```python
from build123d import *

# Parameters (mm, degrees)
BOSS_EXTRUDE1_START         = -2.9464
BOSS_EXTRUDE1_OUTLINE_W     = 230
BOSS_EXTRUDE1_OUTLINE_H     = 101.6
BOSS_EXTRUDE1_OUTLINE_R     = 4
BOSS_EXTRUDE1_OUTLINE_W_2   = 15
BOSS_EXTRUDE1_OUTLINE_H_2   = 91.6
BOSS_EXTRUDE1_DEPTH         = 2.9464
BOSS_EXTRUDE1_START_2       = -101.6
BOSS_EXTRUDE1_2_OUTLINE_W   = 200
BOSS_EXTRUDE1_2_OUTLINE_H   = 101.6
BOSS_EXTRUDE1_2_OUTLINE_R   = 4
BOSS_EXTRUDE1_2_OUTLINE_W_2 = 140
BOSS_EXTRUDE1_2_OUTLINE_H_2 = 40
BOSS_EXTRUDE1_2_DEPTH       = 2.9464
BOSS_EXTRUDE1_START_3       = -98.6536
BOSS_EXTRUDE1_3_OUTLINE_W   = 30
BOSS_EXTRUDE1_3_OUTLINE_H   = 2.9464
BOSS_EXTRUDE1_3_DEPTH       = 95.7072
BOSS_EXTRUDE1_4_OUTLINE_W   = 140
BOSS_EXTRUDE1_4_OUTLINE_H   = 2.9464
BOSS_EXTRUDE1_4_DEPTH       = 17.8536
BOSS_EXTRUDE1_START_4       = -20.8
BOSS_EXTRUDE1_5_OUTLINE_W   = 140
BOSS_EXTRUDE1_5_OUTLINE_H   = 2.9464
BOSS_EXTRUDE1_5_DEPTH       = 17.8536
BOSS_EXTRUDE1_START_5       = -2.95
BOSS_EXTRUDE1_6_DEPTH       = 0.0036
BOSS_EXTRUDE1_START_6       = -50.8
BOSS_EXTRUDE1_7_OUTLINE_R   = 4
BOSS_EXTRUDE1_7_DEPTH       = 101.6
SKETCH3_W                   = 30
SKETCH3_H                   = 2.95
SKETCH3_W_2                 = 30.067744433
BOSS_EXTRUDE2_DEPTH         = 15
CUT_EXTRUDE1_REACH          = 232.007
SKETCH4_W                   = 30
SKETCH4_H                   = 40
FILLET1_R                   = 5
FILLET2_R                   = 5
FILLET3_R                   = 5
FILLET4_R                   = 5


with BuildPart() as part:
    # Boss-Extrude1: read off the stored shape, not the designer's step
    # Boss-Extrude1 outline → Boss-Extrude1 (new body)
    with BuildSketch(Plane.XY.offset(50.8).offset(BOSS_EXTRUDE1_START)):
        with Locations((-85, 0)):
            Rectangle(BOSS_EXTRUDE1_OUTLINE_W, BOSS_EXTRUDE1_OUTLINE_H)
        with Locations((-20, 33.4)):
            Circle(BOSS_EXTRUDE1_OUTLINE_R, mode=Mode.SUBTRACT)
        with Locations((-180, 33.4)):
            Circle(BOSS_EXTRUDE1_OUTLINE_R, mode=Mode.SUBTRACT)
        with Locations((7.5, 0)):
            Rectangle(BOSS_EXTRUDE1_OUTLINE_W_2, BOSS_EXTRUDE1_OUTLINE_H_2, mode=Mode.SUBTRACT)
        with Locations((-180, -33.4)):
            Circle(BOSS_EXTRUDE1_OUTLINE_R, mode=Mode.SUBTRACT)
        with Locations((-20, -33.4)):
            Circle(BOSS_EXTRUDE1_OUTLINE_R, mode=Mode.SUBTRACT)
    extrude(amount=BOSS_EXTRUDE1_DEPTH)



with BuildPart() as body_2:
    # Boss-Extrude1 2 outline → Boss-Extrude1 2 (new body)
    with BuildSketch(Plane.XY.offset(50.8).offset(BOSS_EXTRUDE1_START_2)):
        with Locations((-100, 0)):
            Rectangle(BOSS_EXTRUDE1_2_OUTLINE_W, BOSS_EXTRUDE1_2_OUTLINE_H)
        with Locations((-20, 33.4)):
            Circle(BOSS_EXTRUDE1_2_OUTLINE_R, mode=Mode.SUBTRACT)
        with Locations((-180, 33.4)):
            Circle(BOSS_EXTRUDE1_2_OUTLINE_R, mode=Mode.SUBTRACT)
        with Locations((-180, -33.4)):
            Circle(BOSS_EXTRUDE1_2_OUTLINE_R, mode=Mode.SUBTRACT)
        with Locations((-100, 0)):
            Rectangle(BOSS_EXTRUDE1_2_OUTLINE_W_2, BOSS_EXTRUDE1_2_OUTLINE_H_2, mode=Mode.SUBTRACT)
        with Locations((-20, -33.4)):
            Circle(BOSS_EXTRUDE1_2_OUTLINE_R, mode=Mode.SUBTRACT)
    extrude(amount=BOSS_EXTRUDE1_2_DEPTH)


with BuildPart() as part_1:
    add(part.part)

    add(body_2.part)  # Boss-Extrude1 3 merges body 2
    # Boss-Extrude1 3 outline → Boss-Extrude1 3 (add)
    with BuildSketch(Plane.XY.offset(50.8).offset(BOSS_EXTRUDE1_START_3)):
        with Locations((-15, -49.3268)):
            Rectangle(BOSS_EXTRUDE1_3_OUTLINE_W, BOSS_EXTRUDE1_3_OUTLINE_H)
        with Locations((-185, -49.3268)):
            Rectangle(BOSS_EXTRUDE1_3_OUTLINE_W, BOSS_EXTRUDE1_3_OUTLINE_H)
        with Locations((-15, 49.3268)):
            Rectangle(BOSS_EXTRUDE1_3_OUTLINE_W, BOSS_EXTRUDE1_3_OUTLINE_H)
        with Locations((-185, 49.3268)):
            Rectangle(BOSS_EXTRUDE1_3_OUTLINE_W, BOSS_EXTRUDE1_3_OUTLINE_H)
    extrude(amount=BOSS_EXTRUDE1_3_DEPTH)

    # Boss-Extrude1 4 outline → Boss-Extrude1 4 (add)
    with BuildSketch(Plane.XY.offset(50.8).offset(BOSS_EXTRUDE1_START_3)):
        with Locations((-100, -49.3268)):
            Rectangle(BOSS_EXTRUDE1_4_OUTLINE_W, BOSS_EXTRUDE1_4_OUTLINE_H)
        with Locations((-100, 49.3268)):
            Rectangle(BOSS_EXTRUDE1_4_OUTLINE_W, BOSS_EXTRUDE1_4_OUTLINE_H)
    extrude(amount=BOSS_EXTRUDE1_4_DEPTH)

    # Boss-Extrude1 5 outline → Boss-Extrude1 5 (add)
    with BuildSketch(Plane.XY.offset(50.8).offset(BOSS_EXTRUDE1_START_4)):
        with Locations((-100, -49.3268)):
            Rectangle(BOSS_EXTRUDE1_5_OUTLINE_W, BOSS_EXTRUDE1_5_OUTLINE_H)
        with Locations((-100, 49.3268)):
            Rectangle(BOSS_EXTRUDE1_5_OUTLINE_W, BOSS_EXTRUDE1_5_OUTLINE_H)
    extrude(amount=BOSS_EXTRUDE1_5_DEPTH)

    # Boss-Extrude1 6 outline → Boss-Extrude1 6 (add)
    with BuildSketch(Plane.XY.offset(50.8).offset(BOSS_EXTRUDE1_START_5)):
        Polygon((0, -45.8), (0, -50.8), (30, -50.8), (30, 50.8), (0, 50.8), (0, 45.8), (15, 45.8), (15, -45.8), align=None)
    extrude(amount=BOSS_EXTRUDE1_6_DEPTH)

    # Boss-Extrude1 7 outline → Boss-Extrude1 7 (cut)
    with BuildSketch(Plane(origin=(0, 0, 0), x_dir=(1, 0, 0), z_dir=(0, 1, 0)).offset(BOSS_EXTRUDE1_START_6)):
        with Locations((-190, 33.4)):
            Circle(BOSS_EXTRUDE1_7_OUTLINE_R)
        with Locations((-190, -33.4)):
            Circle(BOSS_EXTRUDE1_7_OUTLINE_R)
        with Locations((-10, 33.4)):
            Circle(BOSS_EXTRUDE1_7_OUTLINE_R)
        with Locations((-10, -33.4)):
            Circle(BOSS_EXTRUDE1_7_OUTLINE_R)
    extrude(amount=BOSS_EXTRUDE1_7_DEPTH, mode=Mode.SUBTRACT)

    # Sketch3 → Boss-Extrude2 (add)
    with BuildSketch(Plane(origin=(0, 0, 47.85), x_dir=(-1, 0, 0), z_dir=(0, 0, -1))):
        with Locations((-15, -49.325)):
            Rectangle(SKETCH3_W, SKETCH3_H)
        with Locations((-15.033872217, 49.325)):
            Rectangle(SKETCH3_W_2, SKETCH3_H)
    extrude(amount=BOSS_EXTRUDE2_DEPTH)

    # Sketch4 → Cut-Extrude1 (cut, up to next)
    with BuildSketch(Plane.XY.offset(50.8), mode=Mode.PRIVATE) as cut_extrude1_sk1:
        with Locations((-170, 0)):
            Rectangle(SKETCH4_W, SKETCH4_H)
    cut_extrude1_tool1 = extrude(cut_extrude1_sk1.sketch, amount=-CUT_EXTRUDE1_REACH, mode=Mode.PRIVATE) & part_1.part
    add(cut_extrude1_tool1.solids().sort_by_distance((-170, 0, 50.8))[0], mode=Mode.SUBTRACT)

    # Fillet1
    fillet1_edges = [part_1.edges().sort_by_distance(p)[0] for p in [
        (-155, -20, 49.3268),
    ]]
    fillet(fillet1_edges, radius=FILLET1_R)

    # Fillet2
    fillet2_edges = [part_1.edges().sort_by_distance(p)[0] for p in [
        (-155, 20, 49.3268),
    ]]
    fillet(fillet2_edges, radius=FILLET2_R)

    # Fillet3
    fillet3_edges = [part_1.edges().sort_by_distance(p)[0] for p in [
        (-185, -20, 49.3268),
    ]]
    fillet(fillet3_edges, radius=FILLET3_R)

    # Fillet4
    fillet4_edges = [part_1.edges().sort_by_distance(p)[0] for p in [
        (-185, 20, 49.3268),
    ]]
    fillet(fillet4_edges, radius=FILLET4_R)


solid = part_1.part
```
Build history of the part. All positions in model axes, mm. A direction names the side the tool comes from. Coordinates: 2 decimals unless noted, no trailing zeros. Order: outer loops, then holes, each group sorted by start corner. A loop starts at its lowest first (then second) coordinate and runs counter-clockwise, first axis right, second up.
Item 1: Mould opens along Y. For faces 6 (the cylindrical face through (-186.185, 49.306, -34.601)), 7 (the flat face through (-83, 50.8, 33)), 8 (the cylindrical face through (-20.867, 29.495, -49.347)) say: released by +Y, released by -Y, zero draft, split by the parting line, or undercut.
Filled in:
face 6: zero draft
face 7: released by +Y
face 8: undercut
Item 2: Saw through at B-B on z = -41. List the corners of the cut face in (x, y).
Filled in:
outline: (-200, -50.8) - (0, -50.8) - (0, -47.85) - (-200, -47.85) - close; (-200, 47.85) - (0, 47.85) - (0, 50.8) - (-200, 50.8) - close
Item 3: Drill centre lines: L1, parallel to Z at x = -190, y = 48.7; L2, parallel to X at y = -49.75, z = 33.4; L3, parallel to X at y = -33, z = -49. Where is each one in solid material? Low to high.
Filled in:
L1: z = -50.8 to -37.4, -29.4 to 29.4, 37.4 to 50.8
L2: x = -200 to -194, -186 to -14, -6 to 30
L3: x = -200 to -183.98, -176.02 to -23.98, -16.02 to 0
Item 4: Saw through at D-D on z = 17.5. List the corners of the cut face in (x, y), then the cut area to 3 significant figures.
Filled in:
outline: (-200, -50.8) - (-170, -50.8) - (-170, -47.85) - (-200, -47.85) - close; (-200, 47.85) - (-170, 47.85) - (-170, 50.8) - (-200, 50.8) - close; (-30, -50.8) - (0, -50.8) - (0, -47.85) - (-30, -47.85) - close; (-30, 47.85) - (0, 47.85) - (0, 50.8) - (-30, 50.8) - close
area: 354 mm2
Item 5: Tool access for faces 1 (the cylindrical face through (-157, -19, 49)), 2 (the flat face through (15, -47.85, 40)), 3 (the flat face through (0, 0, -49)), 4 (the flat face through (-101, -47.854, -33)), 5 (the cylindrical face through (-10.867, -49.347, 37.305)): list every direction of +Z, -Z, +X, -X, +Y, -Y with a clear straight run to the whole face (end or side of a thin tool).
Filled in:
face 1: +Z, -Z
face 2: -Z, +X, -X
face 3: -Z, +X, +Y, -Y
face 4: +X, -X
face 5: +Y, -Y
Item 6: Drop flat-ended pins along their axis: pin 1 Ø2.5 at (y, z) = (-7.5, -49.5) entering from +X; pin 2 Ø1.5 at (x, y) = (-131, -5) entering from -Z; pin 3 Ø3 at (y, z) = (10, 50) entering from +X. Give the stop position or say it passes through.
Filled in:
pin 1: stops at x = 0
pin 2: stops at z = 47.85
pin 3: stops at x = 30
Item 7: Saw through at A-A on y = -27. List the corners of the cut face in (x, z), then the cut area to 3 significant figures.
Filled in:
outline: (-200, -50.8) - (0, -50.8) - (0, -47.85) - (-200, -47.85) - close; (-200, 47.85) - (0, 47.85) - (0, 50.8) - (-200, 50.8) - close; (15, 47.85) - (30, 47.85) - (30, 50.8) - (15, 50.8) - close
area: 1,220 mm2
Item 8: Saw through at C-C on x = -2.5. List the corners of the cut face in (y, z).
Filled in:
outline: (-50.8, -50.8) - (50.8, -50.8) - (50.8, 50.8) - (-50.8, 50.8) - close; hole (-47.85, -47.85) - (47.85, -47.85) - (47.85, 47.85) - (-47.85, 47.85) - close
